Here's how the part is built. I have some questions about the finished solid (model axes, mm). Round coordinates to 2 decimals unless told otherwise and drop trailing zeros. Order: outer loops, then holes, each group sorted by start corner. A loop starts at its lowest first (then second) coordinate and runs counter-clockwise, first axis right, second up. Notation, with made-up numbers: (-29.5, 6.25) - (11.5, 6.25) arc R14 cw to (11.5, 23.25) - close; hole circle Ø4 at (-37.75, -35.75). An arc over 180 degrees is marked (long way). Answer as a JSON object with one key per item and string values.
```python
from build123d import *

# Parameters (mm, degrees)
F0_W           = 152.4
F0_H           = 76.2
F1_DEPTH       = 6.35
F3_D           = 8.4328
F3_CSINK_D     = 16.6624
F3_CSINK_ANGLE = 82
F5_D           = 4.4
F5_CSINK_D     = 8.96
F5_CSINK_ANGLE = 90


with BuildPart() as f1:
    # F0 (on Top) → F1 (new body, symmetric)
    with BuildSketch(Plane.XY):
        Rectangle(F0_W, F0_H)
    extrude(amount=F1_DEPTH, both=True)

    # F3 (through all)
    with Locations(Plane.XY.offset(6.35)):
        with Locations((-19.05, 19.05), (19.05, 19.05), (19.05, -19.05), (-19.05, -19.05)):
            CounterSinkHole(F3_D / 2, F3_CSINK_D / 2, counter_sink_angle=F3_CSINK_ANGLE)

    # F5 (through all)
    with Locations(Plane(origin=(0, 0, -6.35), x_dir=(1, 0, 0), z_dir=(0, 0, -1))):
        with Locations((-57.15, 20), (57.15, 20), (57.15, -20), (-57.15, -20)):
            CounterSinkHole(F5_D / 2, F5_CSINK_D / 2, counter_sink_angle=F5_CSINK_ANGLE)


solid = f1.part
```
1. Thinking about a two-plate mould opening in Y: for faces 1 (the face through (16.676, 22.774, 1.846)), 2 (the face through (-23.07, -17.78, -2.42)), 3 (the face through (-1, 38.1, 0)), 4 (the face through (-76.2, -1, 0)), which applies, pulls with the +Y half, pulls with the -Y half, needs draft (parallel to the pull), parting line crosses it, or undercut?
Responses:
{"face 1": "undercut", "face 2": "undercut", "face 3": "pulls with the +Y half", "face 4": "needs draft"}
2. Imagine slicing it at B-B (z = 4.5). Give the number of separate pieces and of enclosed holes in the cut face, plus the area to 3 significant figures.
Responses:
{"separate pieces": "1", "enclosed holes": "8", "area": "11,000 mm2"}
3. Imagine slicing it at A-A (x = 57.15). List the corners of the cut face in (y, z) for me.
Responses:
{"outline": "(-38.1, -6.35) - (-24.48, -6.35) - (-22.2, -4.07) - (-22.2, 6.35) - (-38.1, 6.35) - close; (-17.8, -4.07) - (-15.52, -6.35) - (15.52, -6.35) - (17.8, -4.07) - (17.8, 6.35) - (-17.8, 6.35) - close; (22.2, -4.07) - (24.48, -6.35) - (38.1, -6.35) - (38.1, 6.35) - (22.2, 6.35) - close"}
4. Imagine slicing it at C-C (x = -19.05). List the corners of the cut face in (y, z) for me.
Responses:
{"outline": "(-38.1, -6.35) - (-23.27, -6.35) - (-23.27, 1.62) - (-27.38, 6.35) - (-38.1, 6.35) - close; (-14.83, -6.35) - (14.83, -6.35) - (14.83, 1.62) - (10.72, 6.35) - (-10.72, 6.35) - (-14.83, 1.62) - close; (23.27, -6.35) - (38.1, -6.35) - (38.1, 6.35) - (27.38, 6.35) - (23.27, 1.62) - close"}
5. For P1, Ø7, axis at x = 57.15, y = 20, coming from the +Z side; P2, Ø7, axis at x = 57.15, y = -20, coming from the -Z side; P3, Ø5, axis at x = -57.15, y = -20, coming from the -Z side, each with a flat end and sliding along its axis, tell me the tip position at first contact or that it passes through.
Responses:
{"P1": "z = 6.35", "P2": "z = -5.37", "P3": "z = -4.37"}
6. If I drill on L1, parallel to X at y = -19.05, z = -4.25; L2, parallel to Y at x = 19.5, z = -1.25; L3, parallel to Y at x = 57.15, z = 0.5, over which ranges is the centre line in solid material (lowest first)? Write a range as [from, to].
Responses:
{"L1": "[-76.2, -59.33], [-54.97, -23.27], [-14.83, 14.83], [23.27, 54.97], [59.33, 76.2]", "L2": "[-38.1, -23.24], [-14.86, 14.86], [23.24, 38.1]", "L3": "[-38.1, -22.2], [-17.8, 17.8], [22.2, 38.1]"}
